from build123d import *
from build123d.topology import SkipClean

# Parameters (mm, degrees)
SKETCH1_R                    = 35
SKETCH1_R_2                  = 20
BOSS_EXTRUDE1_DEPTH          = 2
SKETCH2_R                    = 1.75
CUT_EXTRUDE1_DEPTH           = 50.537864306
CIRPATTERN1_COUNT            = 4
BOSS_EXTRUDE2_DEPTH          = 2
CHAMFER1_SIZE                = 2
CIRPATTERN2_COUNT            = 2
CIRPATTERN2_ANGLE            = 90
CHAMFER1_OF_CIRPATTERN2_SIZE = 2
SKETCH5_R                    = 1.5
SKETCH5_W                    = 10
SKETCH5_H                    = 6
CUT_EXTRUDE2_DEPTH           = 50.658836072


with BuildPart() as part:
    # Sketch1 → Boss-Extrude1 (new body)
    with BuildSketch(Plane.XY):
        Circle(SKETCH1_R)
        Circle(SKETCH1_R_2, mode=Mode.SUBTRACT)
    extrude(amount=BOSS_EXTRUDE1_DEPTH)

    # Sketch2 → Cut-Extrude1 (cut, through all)
    with BuildSketch(Plane.XY.offset(2)):
        with Locations((5, 30)):
            Circle(SKETCH2_R)
        with Locations((-5, 30)):
            Circle(SKETCH2_R)
    cut_extrude1 = extrude(amount=-CUT_EXTRUDE1_DEPTH, mode=Mode.SUBTRACT)

    # CirPattern1: Cut-Extrude1 ×4 about axis
    cirpattern1_axis = Axis((0, 0, 0), (0, 0, 1))
    for i in range(1, CIRPATTERN1_COUNT):
        add(cut_extrude1.rotate(cirpattern1_axis, i * 360 / CIRPATTERN1_COUNT), mode=Mode.SUBTRACT)

    # Sketch3 → Boss-Extrude2 (add)
    with SkipClean():  # the faces are left unmerged after this step: merging them gives an invalid solid
        with BuildSketch(Plane.XY.offset(2)):
            with BuildLine():
                Line((-30.130645656, -17.80854268), (17.80854268, 30.130645656))
                ThreePointArc((17.80854268, 30.130645656), (24.748737342, 24.748737342), (30.130645656, 17.80854268))
                Line((30.130645656, 17.80854268), (-17.80854268, -30.130645656))
                ThreePointArc((-17.80854268, -30.130645656), (-24.748737342, -24.748737342), (-30.130645656, -17.80854268))
            make_face()
        boss_extrude2 = extrude(amount=BOSS_EXTRUDE2_DEPTH)

    # Chamfer1
    chamfer1_edges = [part.edges().sort_by_distance(p)[0] for p in [
        (-24.748737342, -24.748737342, 4),
        (24.748737342, 24.748737342, 4),
    ]]
    chamfer(chamfer1_edges, length=CHAMFER1_SIZE - 0.0001)  # a hair under: the kernel refuses the full size

    # CirPattern2: Boss-Extrude2 ×2 about axis
    with SkipClean():  # the faces are left unmerged after this step: merging them gives an invalid solid
        cirpattern2_axis = Axis((0, 0, 0), (0, 0, 1))
        for i in range(1, CIRPATTERN2_COUNT):
            add(boss_extrude2.rotate(cirpattern2_axis, i * CIRPATTERN2_ANGLE / (CIRPATTERN2_COUNT - 1)))

    # Chamfer1 of CirPattern2
    chamfer1_of_cirpattern2_edges = [part.edges().sort_by_distance(p)[0] for p in [
        (24.748737342, -24.748737342, 4),
        (-24.748737342, 24.748737342, 4),
    ]]
    chamfer(chamfer1_of_cirpattern2_edges, length=CHAMFER1_OF_CIRPATTERN2_SIZE - 0.0001)  # a hair under: the kernel refuses the full size

    # Sketch5 → Cut-Extrude2 (cut, through all)
    with BuildSketch(Plane.XY.offset(4)):
        with Locations((0, 8)):
            Circle(SKETCH5_R)
        with Locations((-8, 8)):
            Circle(SKETCH5_R)
        with Locations((-8, 0)):
            Circle(SKETCH5_R)
        with Locations((-8, -8)):
            Circle(SKETCH5_R)
        with Locations((8, -8)):
            Circle(SKETCH5_R)
        with Locations((8, 0)):
            Circle(SKETCH5_R)
        with Locations((8, 8)):
            Circle(SKETCH5_R)
        with Locations((0, -8)):
            Circle(SKETCH5_R)
        with Locations((-16, 8)):
            Circle(SKETCH5_R)
        with Locations((-16, 0)):
            Circle(SKETCH5_R)
        with Locations((-16, -8)):
            Circle(SKETCH5_R)
        with Locations((16, -8)):
            Circle(SKETCH5_R)
        with Locations((16, 0)):
            Circle(SKETCH5_R)
        with Locations((16, 8)):
            Circle(SKETCH5_R)
        Rectangle(SKETCH5_W, SKETCH5_H)
    extrude(amount=-CUT_EXTRUDE2_DEPTH, mode=Mode.SUBTRACT)


solid = part.part
Geometry check sheet. Reference: the model listing, model coordinates, mm. A direction names the side the tool comes from. Give positions to 0.01 mm unless a question says otherwise; leave off trailing zeros. Order: outer loops, then holes, each group sorted by start corner. A loop starts at its lowest first (then second) coordinate and runs counter-clockwise, first axis right, second up. Notation, with made-up numbers: (-6.75, -11.75) - (7.25, -11.75) arc R9 cw to (7.25, -4.75) - close; hole circle Ø1 at (55, 24.25). An arc over 180 degrees is marked (long way). Answer as a JSON object with one key per item and string values.
(1) Tool access check on faces 1 (the flat face through (0, 27, 2)), 2 (the flat face through (-8.78, -21.1, 2.99)), 3 (the flat face through (-21.35, -9.03, 2.99)), 4 (the flat face through (0, -4, 2)). Record the directions out of +Z, -Z, +X, -X, +Y, -Y that give a thin tool (end or side, any length) a straight path to the whole face; none if there is none.
Report:
{"face 1": "+Z, +Y", "face 2": "+Z, -Y", "face 3": "+Z, -X", "face 4": "-Z"}
(2) Draft check along X on faces 5 (the cylindrical face through (-17.5, 8.07, 3.01)), 6 (the flat face through (27, 0, 2)), 7 (the flat face through (21.35, 9.03, 2.99)). Enter one of: released by +X, released by -X, zero draft, split by the parting line, or undercut.
Report:
{"face 5": "undercut", "face 6": "zero draft", "face 7": "released by +X"}
(3) Material ranges on line 1 (Y direction, x = 0, z = 1.55); line 2 (Y direction, x = -3.5, z = 0.2); line 3 (Y direction, x = -8, z = 2.6), recorded low to high.
Report:
{"line 1": "-35 to -20, 20 to 35", "line 2": "-34.82 to -30.9, -29.1 to -19.69, 19.69 to 29.1, 30.9 to 34.82", "line 3": "-20.32 to -9.5, -6.5 to -1.5, 1.5 to 6.5, 9.5 to 20.32"}
(4) Cross-section at A-A (z = 1.3). State how many separate pieces and enclosed holes the cut face has, then the cut area to 3 significant figures.
Report:
{"separate pieces": "1", "enclosed holes": "9", "area": "2,510 mm^2"}
(5) Cross-section at B-B (y = 5). Record the cut outline in (x, z).
Report:
{"outline": "(-34.64, 0) - (-31.75, 0) - (-31.75, 2) - (-34.64, 2) - close; (-28.25, 0) - (-19.36, 0) - (-19.36, 2) - (-28.25, 2) - close; (-17.32, 2) - (17.32, 2) - (17.32, 4) - (-17.32, 4) - close; (19.36, 0) - (28.25, 0) - (28.25, 2) - (19.36, 2) - close; (31.75, 0) - (34.64, 0) - (34.64, 2) - (31.75, 2) - close"}
(6) Cross-section at C-C (x = -8). Record the cut outline in (y, z), then the cut area to 3 significant figures.
Report:
{"outline": "(-34.07, 0) - (-18.33, 0) - (-18.33, 2) - (-9.5, 2) - (-9.5, 4) - (-20.32, 4) - (-20.32, 2) - (-34.07, 2) - close; (-6.5, 2) - (-1.5, 2) - (-1.5, 4) - (-6.5, 4) - close; (1.5, 2) - (6.5, 2) - (6.5, 4) - (1.5, 4) - close; (9.5, 2) - (18.33, 2) - (18.33, 0) - (34.07, 0) - (34.07, 2) - (20.32, 2) - (20.32, 4) - (9.5, 4) - close", "area": "126 mm^2"}
(7) Depth check by flat-ended pin: pin 1 Ø4 at (x, y) = (5, -30) entering from +Z; pin 2 Ø1 at (y, z) = (0.5, 3.5) entering from +X; pin 3 Ø3.5 at (x, y) = (-8, 8) entering from -Z. Enter the tip coordinate at first touch or a pass-through.
Report:
{"pin 1": "z = 2", "pin 2": "x = 13.32", "pin 3": "z = 2"}
